Autodesk Inventor part; units mm, degrees
ref_plane "Work Plane1" through (0, 0, -914.4) normal (0, 0, 1) x (1, 0, 0)
ref_plane "Work Plane2" through (0, -584.2, -1143) normal (0, -1, 0) x (1, 0, 0)
ref_plane "YZ Plane" through (0, 0, 0) normal (1, 0, 0) x (0, 1, 0)
sketch "Sketch1" plane through (0, 0, 0) normal (1, 0, 0) x (0, 1, 0)
  line L0 (0, 0) -> (-1168.4, 0)
  line L1 (-1168.4, 0) -> (-1168.4, -1828.8)
  line L2 (-1168.4, -1828.8) -> (0, -1828.8)
  line L3 (0, -1828.8) -> (0, 0)
  dimension "d0" = 1168.4
  dimension "d1" = 1828.8
extrude "Extrusion1" add sketch "Sketch1" along normal blind 25.4
sketch "Sketch2" plane through (0, -1168.4, -1828.8) normal (0, -1, 0) x (1, 0, 0)
  line L0 (25.4, 1828.8) -> (25.4, 0)
  line L1 (0, 1828.8) -> (0, 0)
  line L2 (25.4, 1600.2) -> (0, 1600.2)
  line L3 (0, 1600.2) -> (0, 1143)
  line L4 (0, 1143) -> (25.4, 1143)
  line L5 (25.4, 1143) -> (25.4, 1600.2)
  line L6 (25.4, 685.8) -> (0, 685.8)
  line L7 (0, 685.8) -> (0, 228.6)
  line L8 (0, 228.6) -> (25.4, 228.6)
  line L9 (25.4, 228.6) -> (25.4, 685.8)
  line L10 (12.7, 1600.2) -> (12.7, 1143)
  line L11 (12.7, 685.8) -> (12.7, 228.6)
  line L12 (0, 1828.8) -> (25.4, 1828.8)
  line L13 (12.7, 1828.8) -> (12.7, 1600.2)
  line L14 (0, 0) -> (25.4, 0)
  line L15 (12.7, 0) -> (12.7, 228.6)
  dimension "d4" = 228.6
  dimension "d5" = 457.2
extrude "Extrusion2" add sketch "Sketch2" along normal blind 50.8 contours L0 L4 L10 L2 | L10 L4 L1 L2 | L0 L8 L11 L6 | L11 L8 L1 L6
sketch "Sketch3" plane through (0, -1168.4, 0) normal (0, 0, 1) x (1, 0, 0)
  line L0 (0, 0) -> (0, 1168.4)
  line L1 (25.4, 0) -> (25.4, 1168.4)
  line L2 (0, 203.2) -> (25.4, 203.2)
  line L3 (25.4, 203.2) -> (25.4, 406.4)
  line L4 (25.4, 406.4) -> (0, 406.4)
  line L5 (0, 406.4) -> (0, 203.2)
  line L6 (0, 1168.4) -> (0, 0)
  line L7 (0, 0) -> (25.4, 0)
  line L8 (25.4, 1168.4) -> (25.4, 0)
  line L9 (0, 1168.4) -> (25.4, 1168.4)
  line L10 (0, 965.2) -> (25.4, 965.2)
  line L11 (25.4, 965.2) -> (25.4, 762)
  line L12 (25.4, 762) -> (0, 762)
  line L13 (0, 762) -> (0, 965.2)
  dimension "d8" = 203.2
  dimension "d9" = 203.2
  dimension "d12" = 203.2
  dimension "d13" = 355.6
extrude "Extrusion3" add sketch "Sketch3" along normal blind 25.4 contours L0 L4 L1 L2 | L0 L10 L1 L12
ref_plane "Work Plane1" through (0, 0, -914.4) normal (0, 0, 1) x (1, 0, 0)
mirror "Mirror1" about plane through (0, 0, -914.4) normal (0, 0, 1) of "Extrusion3"
ref_plane "Work Plane2" through (0, -584.2, -1143) normal (0, -1, 0) x (1, 0, 0)
mirror "Mirror2" about plane through (0, -584.2, -1143) normal (0, -1, 0) of "Extrusion2"
properties part number "rev1 large wall"
Check sheet for the modelled part. Datum: model origin and axes. Units: mm. Round coordinates to 2 decimals unless told otherwise and drop trailing zeros. Write each loop counter-clockwise with the first axis right and the second up, starting at its lowest first coordinate (ties: lowest second). Pieces come first, ordered by that corner, then holes. Notation, with made-up numbers: (-26.75, 19) -> (-21.75, 19) arc R14 ccw to (-21.75, 46) -> close; hole circle Ø1 at (-17, -19.5). An arc over 180 degrees is marked (long way). Put each result on its own line as item: value.
(1) Sectioned sample at B-B (z = -1651). Enter the section's corners in (x, y), plus the area to 3 significant figures.
Values found:
outline: (0, -1168.4) -> (25.4, -1168.4) -> (25.4, 0) -> (0, 0) -> close
area: 29,700 mm^2
(2) Go/stop test with flat-tipped pins: pin 1 Ø7.5 at (x, z) = (12.5, -1844.5) entering from -Y; pin 2 Ø7.5 at (x, z) = (12.5, 10) entering from +Y; pin 3 Ø7.5 at (x, z) = (11.5, -169) entering from +Y. Record where each tip stops, or that it passes through.
Values found:
pin 1: stops at y = -965.2
pin 2: stops at y = -203.2
pin 3: stops at y = 0
(3) Sectioned sample at A-A (y = -442.5). Enter the section's corners in (x, z).
Values found:
outline: (0, -1828.8) -> (25.4, -1828.8) -> (25.4, 0) -> (0, 0) -> close
(4) Material ranges on line 1 (Y direction, x = 11, z = -1023.5); line 2 (Z direction, x = 20, y = -175), recorded low to high.
Values found:
line 1: y = -1168.4 to 0
line 2: z = -1828.8 to 0
